```python
from build123d import *

# Parameters (mm, degrees)
SKETCH4_R           = 4.7625
SKETCH4_R_2         = 1.5875
BOSS_EXTRUDE1_DEPTH = 12.7
CUT_EXTRUDE3_DEPTH  = 3.175
CUT_EXTRUDE2_DEPTH  = 3.175
SKETCH8_R           = 2.38125
CUT_EXTRUDE4_DEPTH  = 3.175
FILLET1_R           = 0.396875
CHAMFER1_SIZE       = 0.254


with BuildPart() as part:
    # Sketch4 → Boss-Extrude1 (new body)
    with BuildSketch(Plane(origin=(0, 0, 0), x_dir=(1, 0, 0), z_dir=(0, 1, 0))):
        Circle(SKETCH4_R)
        Circle(SKETCH4_R_2, mode=Mode.SUBTRACT)
    extrude(amount=BOSS_EXTRUDE1_DEPTH)

    # Sketch7 → Cut-Extrude3 (cut)
    with BuildSketch(Plane.XZ):
        Polygon((1.624115175, 2.81305), (-1.624115175, 2.81305), (-3.248230349, 0), (-1.624115175, -2.81305), (1.624115175, -2.81305), (3.248230349, 0), align=None)
    extrude(amount=-CUT_EXTRUDE3_DEPTH, mode=Mode.SUBTRACT)

    # Sketch6 → Cut-Extrude2 (cut)
    with BuildSketch(Plane(origin=(0, 12.7, 0), x_dir=(1, 0, 0), z_dir=(0, 1, 0))):
        Polygon((1.833087105, 3.175), (-1.833087105, 3.175), (-3.666174209, 0), (-1.833087105, -3.175), (1.833087105, -3.175), (3.666174209, 0), align=None)
    extrude(amount=-CUT_EXTRUDE2_DEPTH, mode=Mode.SUBTRACT)

    # Sketch8 → Cut-Extrude4 (cut)
    with BuildSketch(Plane(origin=(0, 9.525, 0), x_dir=(1, 0, 0), z_dir=(0, 1, 0))):
        Circle(SKETCH8_R)
    extrude(amount=-CUT_EXTRUDE4_DEPTH, mode=Mode.SUBTRACT)

    # Fillet1
    fillet1_edges = [part.edges().sort_by_distance(p)[0] for p in [
        (2.436172762, 3.175, 1.406525),
        (1.624115175, 1.5875, 2.81305),
        (2.436172762, 3.175, -1.406525),
        (3.248230349, 1.5875, 0),
        (0, 3.175, -2.81305),
        (1.624115175, 1.5875, -2.81305),
        (-2.436172762, 3.175, -1.406525),
        (-1.624115175, 1.5875, -2.81305),
        (-2.436172762, 3.175, 1.406525),
        (-3.248230349, 1.5875, 0),
        (0, 3.175, 2.81305),
        (-1.624115175, 1.5875, 2.81305),
        (2.749630657, 9.525, -1.5875),
        (1.833087105, 11.1125, -3.175),
        (2.749630657, 9.525, 1.5875),
        (3.666174209, 11.1125, 0),
        (0, 9.525, 3.175),
        (1.833087105, 11.1125, 3.175),
        (-2.749630657, 9.525, 1.5875),
        (-1.833087105, 11.1125, 3.175),
        (-2.749630657, 9.525, -1.5875),
        (-3.666174209, 11.1125, 0),
        (0, 9.525, -3.175),
        (-1.833087105, 11.1125, -3.175),
        (-2.38125, 6.35, 0),
    ]]
    fillet(fillet1_edges, radius=FILLET1_R)

    # Chamfer1
    chamfer1_edges = [part.edges().sort_by_distance(p)[0] for p in [
        (-1.5875, 3.175, 0),
        (-4.7625, 0, 0),
        (-4.7625, 12.7, 0),
        (-1.5875, 6.35, 0),
        (-2.38125, 9.525, 0),
        (2.436172762, 0, 1.406525),
        (2.436172762, 0, -1.406525),
        (0, 0, -2.81305),
        (-2.436172762, 0, -1.406525),
        (-2.436172762, 0, 1.406525),
        (0, 0, 2.81305),
        (0, 12.7, -3.175),
        (2.749630657, 12.7, -1.5875),
        (-2.749630657, 12.7, 1.5875),
        (-2.749630657, 12.7, -1.5875),
        (0, 12.7, 3.175),
        (2.749630657, 12.7, 1.5875),
        (3.186833573, 0, 0),
        (-1.593416787, 0, -2.759878832),
        (-3.186833573, 0, 0),
        (-1.593416787, 0, 2.759878832),
        (1.593416787, 0, 2.759878832),
        (1.593416787, 0, -2.759878832),
        (1.802388717, 12.7, -3.121828832),
        (-3.604777433, 12.7, 0),
        (-1.802388717, 12.7, 3.121828832),
        (1.802388717, 12.7, 3.121828832),
        (3.604777433, 12.7, 0),
        (-1.802388717, 12.7, -3.121828832),
    ]]
    chamfer(chamfer1_edges, length=CHAMFER1_SIZE)


solid = part.part
```
The listing builds one solid part. Answer for the finished solid, in the listing's coordinates (mm). A direction names the side the tool comes from. Give positions to 0.01 mm unless a question says otherwise; leave off trailing zeros. Order: outer loops, then holes, each group sorted by start corner. A loop starts at its lowest first (then second) coordinate and runs counter-clockwise, first axis right, second up.
1) Given P1, Ø1.3, axis at x = 1, y = 11, coming from the +Z side; P2, Ø5.5, axis at x = 0, z = 0, coming from the +Y side (3 decimals); P3, Ø3, axis at x = 0, z = 0, coming from the +Y side; P4, Ø4, axis at x = 0.5, z = 1, coming from the -Y side, each flat-ended and moving along its own axis, determine where each tip first touches the part or whether it passes through.
Reported:
P1: stops at z = 4.75
P2: stops at y = 9.525
P3: passes through
P4: stops at y = 0.07
2) For faces 4 (the face through (-3.1, 0, -1.1)), 5 (the face through (0, 11, 3.175)), 6 (the face through (-2.348, 3.056, 1.333)), determine the directions among +Z, -Z, +X, -X, +Y, -Y from which every point of the face is accessible in a straight line to the end or side of a thin tool.
Reported:
face 4: +Z, -Z, +X, -X, -Y
face 5: +Y
face 6: -Y
3) Find section C-C on y = 5.75. Write down the section's boundary in (x, z) (1 decimal), then the cut area to 3 significant figures.
Reported:
outline: circle Ø9.5 at (0, 0); hole circle Ø3.2 at (0, 0)
area: 63.3 mm2
4) Determine the mould class of faces 1 (the face through (3, 12.7, -2)), 2 (the face through (2, 3.175, 0)), 3 (the face through (0, 1, -2.813)) for opening direction Z: pulls with the +Z half, pulls with the -Z half, needs draft (parallel to the pull), parting line crosses it, or undercut.
Reported:
face 1: needs draft
face 2: undercut
face 3: undercut
5) Consider line 1 along Z through (x, y) = (0, 4.95); line 2 along X through (y, z) = (8.7, 0). Determine where each line is inside the solid, lowest interval first.
Reported:
line 1: z = -4.76 to -1.59, 1.59 to 4.76
line 2: x = -4.76 to -2.38, 2.38 to 4.76
